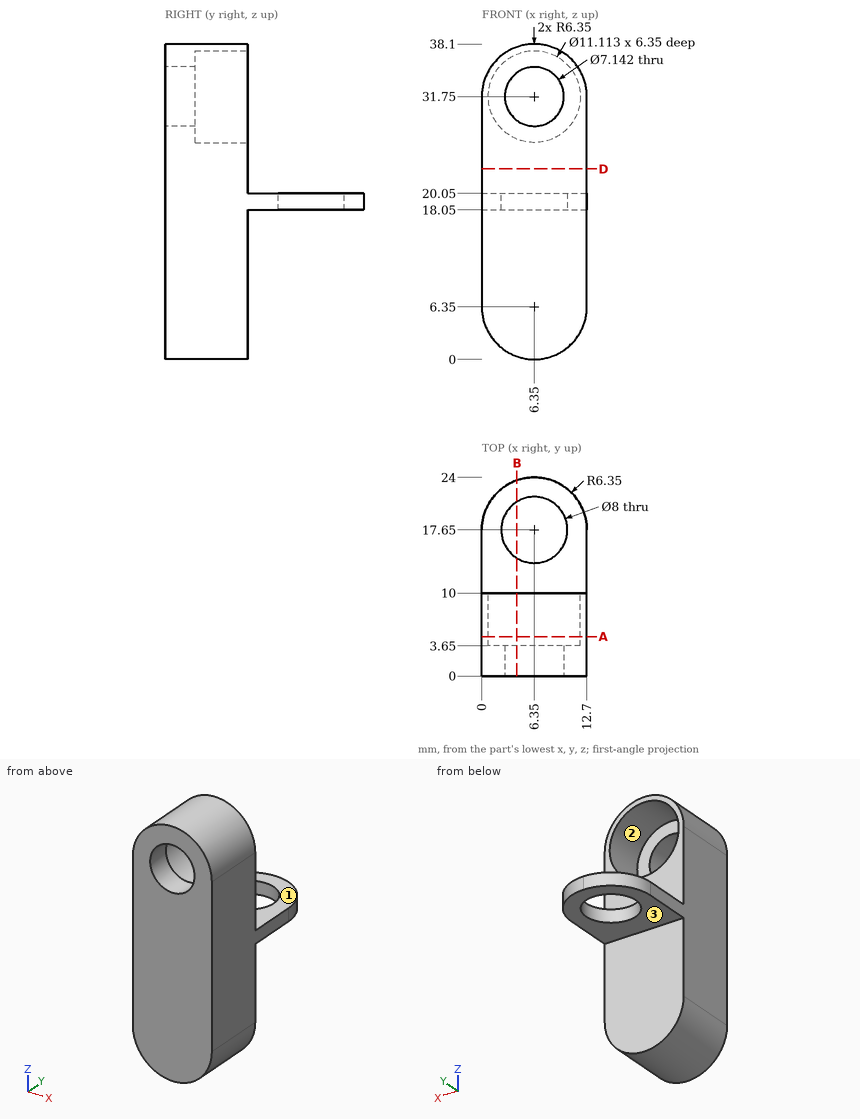
Here's the drawing with two shaded views (mm, measured from the low corner). I have some questions. A direction names the side the tool comes from. Round coordinates to 2 decimals unless told otherwise and drop trailing zeros. Order: outer loops, then holes, each group sorted by start corner. A loop starts at its lowest first (then second) coordinate and runs counter-clockwise, first axis right, second up. Notation, with made-up numbers: (30, 69) -> (38, 69) arc R21 ccw to (38, 96) -> close; hole circle Ø7 at (-21, -12). An arc over 180 degrees is marked (long way). Use a Markdown table: item, result. Add a question column.
(1) For pin 1 Ø4 at (y, z) = (19.5, 23) entering from -X; pin 2 Ø5.5 at (x, z) = (8.5, 30.5) entering from +Y, each with a flat end and sliding along its axis, tell me the tip position at first contact or that it passes through.
(2) Suppose I cut it at A-A, the plane y = 4.75. Please give me the cut outline in (x, z), and give its area (3 significant figures).
(3) Suppose I cut it at B-B, the plane x = 4.25. Count the separate pieces of the cut face and the enclosed holes in it, and give its area (3 significant figures).
(4) For the marked faces 1, 2 and 3, which set-ups out of +Z, -Z, +X, -X, +Y, -Y let a thin tool reach every point of the face, with its end or its side?
(5) Suppose I cut it at D-D, the plane z = 23. Please give me the cut outline in (x, y), and give its area (3 significant figures).
(6) I need wall thicknesses on line 1 along X through (y, z) = (6, 31.5); line 2 along Y through (x, z) = (7.5, 8); line 3 along Z through (x, y) = (9, 21.5). Which ranges of each line are inside material? Lowest first, please.
Verdict:
| question | item | result |
|---|---|---|
| 1 | pin 1 | through |
| 1 | pin 2 | y = 3.65 |
| 2 | outline | (0, 6.35) arc R6.35 ccw to (12.7, 6.35) -> (12.7, 31.75) arc R6.35 ccw to (0, 31.75) -> close; hole circle Ø11.11 at (6.35, 31.75) |
| 2 | area | 352 mm2 |
| 3 | separate pieces | 3 |
| 3 | enclosed holes | 0 |
| 3 | area | 301 mm2 |
| 4 | face 1 | +Z, +X, -X, +Y |
| 4 | face 2 | +Y |
| 4 | face 3 | -Z, +X, -X, +Y |
| 5 | outline | (0, 0) -> (12.7, 0) -> (12.7, 10) -> (0, 10) -> close |
| 5 | area | 127 mm2 |
| 6 | line 1 | 0 to 0.8, 11.9 to 12.7 |
| 6 | line 2 | 0 to 10 |
| 6 | line 3 | 18.05 to 20.05 |
